Read the model definition and answer for the solid it produces. Units are mm, in the model's axes. A direction names the side the tool comes from. Give positions to 0.01 mm unless a question says otherwise; leave off trailing zeros. Order: outer loops, then holes, each group sorted by start corner. A loop starts at its lowest first (then second) coordinate and runs counter-clockwise, first axis right, second up.
Item 1: A cutting plane is placed at C-C (y = -1). State how many separate pieces and enclosed holes the cut face has, plus the area to 3 significant figures.
Item 2: Which of the six approach directions +Z, -Z, +X, -X, +Y, -Y give full straight-line access (tool end or side, diameter ignored) to faces 1 (the face through (34.591, -1.252, 26.958)), 2 (the face through (16, -2.54, -16))?
Item 3: A cutting plane is placed at A-A (z = 0). Write down the section's boundary in (x, y).
Item 4: Given pin 1 Ø1.5 at (x, y) = (5.5, -0.5) entering from -Z; pin 2 Ø1.5 at (y, z) = (-1, 34.5) entering from +X, each flat-ended and moving along its own axis, determine where each tip first touches the part or whether it passes through.
Item 5: A cutting plane is placed at B-B (x = -13.5). Write down the section's boundary in (y, z), plus the area to 3 significant figures.
Item 6: The mould has two halves that part along Z. Classify faces 3 (the face through (14.555, -1.252, -21.54)), 4 (the face through (16, 0, -16)): +Z half, -Z half, draft (parallel to the pull), parting line (faces both ways), or undercut.
Item 7: A cutting plane is placed at D-D (x = 53.5). Write down the section's boundary in (y, z).
Item 8: Find the intervals of material crossed by line 1 along X through (y, z) = (-0.9, 1); line 2 along X through (y, z) = (-1.5, -9) (3 decimals); line 3 along X through (y, z) = (-2.2, 12.5), in increasing order.
from build123d import *

# Parameters (mm, degrees)
F1_R     = 76.2
F1_R_2   = 17.9959
F2_DEPTH = 2.54
F0_D     = 5.0038


with BuildPart() as f2:
    # F1 (on Front) → F2 (new body)
    with BuildSketch(Plane.XZ):
        Circle(F1_R)
        with BuildLine():
            Line((-38.44313, -50.540833), (-18.178202, -18.584719))
            ThreePointArc((-18.178202, -18.584719), (-11.270308, -23.426886), (-3.175655, -25.80221))
            Line((-3.175655, -25.80221), (15.538346, -61.569553))
            ThreePointArc((15.538346, -61.569553), (-12.710839, -62.214826), (-38.44313, -50.540833))
        make_face(mode=Mode.SUBTRACT)
        with BuildLine():
            Line((-62.99121, 8.02231), (-25.18394, 6.450426))
            ThreePointArc((-25.18394, 6.450426), (-25.923432, -1.95307), (-23.933196, -10.150907))
            Line((-23.933196, -10.150907), (-45.551624, -44.241379))
            ThreePointArc((-45.551624, -44.241379), (-60.235039, -20.099503), (-62.99121, 8.02231))
        make_face(mode=Mode.SUBTRACT)
        with BuildLine():
            Line((24.54808, -58.563143), (7.005737, -25.035144))
            ThreePointArc((7.005737, -25.035144), (14.653124, -21.473816), (20.757542, -15.651302))
            Line((20.757542, -15.651302), (61.08997, -17.328174))
            ThreePointArc((61.08997, -17.328174), (47.5242, -42.115323), (24.54808, -58.563143))
        make_face(mode=Mode.SUBTRACT)
        with BuildLine():
            ThreePointArc((-61.08997, 17.328174), (-47.5242, 42.115323), (-24.54808, 58.563143))
            Line((-24.54808, 58.563143), (-7.005737, 25.035144))
            ThreePointArc((-7.005737, 25.035144), (-14.653124, 21.473816), (-20.757542, 15.651302))
            Line((-20.757542, 15.651302), (-61.08997, 17.328174))
        make_face(mode=Mode.SUBTRACT)
        Circle(F1_R_2, mode=Mode.SUBTRACT)
        with BuildLine():
            Line((62.99121, -8.02231), (25.18394, -6.450426))
            ThreePointArc((25.18394, -6.450426), (25.923432, 1.95307), (23.933196, 10.150907))
            Line((23.933196, 10.150907), (45.551624, 44.241379))
            ThreePointArc((45.551624, 44.241379), (60.235039, 20.099503), (62.99121, -8.02231))
        make_face(mode=Mode.SUBTRACT)
        with BuildLine():
            ThreePointArc((18.178202, 18.584719), (11.270308, 23.426886), (3.175655, 25.80221))
            Line((3.175655, 25.80221), (-15.538346, 61.569553))
            ThreePointArc((-15.538346, 61.569553), (12.710839, 62.214826), (38.44313, 50.540833))
            Line((38.44313, 50.540833), (18.178202, 18.584719))
        make_face(mode=Mode.SUBTRACT)
    extrude(amount=F2_DEPTH)

    # F0 (through all)
    with Locations(Plane(origin=(0, 0, 0), x_dir=(1, 0, 0), z_dir=(0, 1, 0))):
        with Locations((19.049441, 10.9982), (19.049441, -10.9982), (0, -21.9964), (-19.049441, -10.9982), (-19.049441, 10.9982), (0, 21.9964)):
            Hole(F0_D / 2)


solid = f2.part
Response values:
1. separate pieces: 1
1. enclosed holes: 13
1. area: 8,750 mm2
2. face 1: +Y, -Y
2. face 2: +Z, -Z, +X, -X, -Y
3. outline: (-76.2, -2.54) - (-63.5, -2.54) - (-63.5, 0) - (-76.2, 0) - close; (-26, -2.54) - (-18, -2.54) - (-18, 0) - (-26, 0) - close; (18, -2.54) - (26, -2.54) - (26, 0) - (18, 0) - close; (63.5, -2.54) - (76.2, -2.54) - (76.2, 0) - (63.5, 0) - close
4. pin 1: stops at z = -76.05
4. pin 2: stops at x = 68.32
5. outline: (-2.54, -74.99) - (0, -74.99) - (0, -62.05) - (-2.54, -62.05) - close; (-2.54, -22.22) - (0, -22.22) - (0, -11.9) - (-2.54, -11.9) - close; (-2.54, 11.9) - (0, 11.9) - (0, 22.22) - (-2.54, 22.22) - close; (-2.54, 37.45) - (0, 37.45) - (0, 57.67) - (-2.54, 57.67) - close; (-2.54, 62.05) - (0, 62.05) - (0, 74.99) - (-2.54, 74.99) - close
5. area: 170 mm2
6. face 3: undercut
6. face 4: draft
7. outline: (-2.54, -54.26) - (0, -54.26) - (0, -34.21) - (-2.54, -34.21) - close; (-2.54, -17.01) - (0, -17.01) - (0, -7.63) - (-2.54, -7.63) - close; (-2.54, 34.21) - (0, 34.21) - (0, 54.26) - (-2.54, 54.26) - close
8. line 1: x = -76.19 to -63.49, -25.98 to -17.97, 17.97 to 25.98, 63.49 to 76.19
8. line 2: x = -75.667 to -62.859, -24.389 to -20.555, -17.544 to -15.584, 15.584 to 17.544, 20.555 to 75.667
8. line 3: x = -75.17 to -21.05, -17.05 to -12.95, 12.95 to 17.05, 21.05 to 25.42, 62.26 to 75.17
